from build123d import *

# Parameters (mm, degrees)
CORTAR_EXTRUIR1_DEPTH = 15


with BuildPart() as part:
    # Croquis1 → Revolución1 (revolve)
    with BuildSketch(Plane(origin=(0, 0, 0), x_dir=(0, 0, -1), z_dir=(1, 0, 0))):
        Polygon((40, 10), (0, 10), (0, -10), (40, -10), (40, -4.682903261), (36.75, -3.5), (36.75, 3.5), (40, 4.682903261), align=None)
    revolve(axis=Axis((0, 0, 0), (0, 1, 0)))

    # Croquis2 → Cortar-Extruir1 (cut, symmetric)
    with BuildSketch(Plane(origin=(0, 0, 0), x_dir=(1, 0, 0), z_dir=(0, 1, 0))):
        with BuildLine():
            Line((3, 2.645751311), (3, -2.645751311))
            ThreePointArc((3, -2.645751311), (-4, 0), (3, 2.645751311))
        make_face()
    extrude(amount=CORTAR_EXTRUIR1_DEPTH, both=True, mode=Mode.SUBTRACT)


solid = part.part
The model under review builds one solid part; all positions refer to its coordinate system, in mm. A direction names the side the tool comes from. Round coordinates to 2 decimals unless told otherwise and drop trailing zeros. Order: outer loops, then holes, each group sorted by start corner. A loop starts at its lowest first (then second) coordinate and runs counter-clockwise, first axis right, second up. Notation, with made-up numbers: (1, 27.5) - (33, 27.5) arc R6 ccw to (33, 31.5) - close; hole circle Ø2 at (17.25, -12). An arc over 180 degrees is marked (long way). Use one line per item in the form item = value.
Q1. Add section D-D on y = -1.5. Give the boundary of the cut face in (x, z), then the cut area to 3 significant figures.
Response values:
outline = circle Ø73.5 at (0, 0); hole (3, -2.65) - (3, 2.65) arc R4 ccw (long way) to start
area = 4,200 mm^2
Q2. Tool access review of faces 4 (the flat face through (-1, -10, 8)), 5 (the cylindrical face through (35.876, 0.049, 7.967)), 6 (the flat face through (3, 0, 0)): name each direction out of +Z, -Z, +X, -X, +Y, -Y from which nothing blocks a thin tool from reaching the whole face with its end or side.
Response values:
face_4 = +Z, -Z, +X, -X, -Y
face_5 = none
face_6 = +Y, -Y
Q3. To check wall thickness, follow line 1 (Z direction, x = 0, y = -5.5); line 2 (X direction, y = 5, z = 0); line 3 (X direction, y = 2, z = 0). State the ranges of each line that lie inside material, in increasing order.
Response values:
line_1 = -40 to -4, 4 to 40
line_2 = -40 to -4, 3 to 40
line_3 = -36.75 to -4, 3 to 36.75
Q4. Add section C-C on y = 8. Give the boundary of the cut face in (x, z).
Response values:
outline = circle Ø80 at (0, 0); hole (3, -2.65) - (3, 2.65) arc R4 ccw (long way) to start
Q5. Add section B-B on x = 0. Give the boundary of the cut face in (y, z).
Response values:
outline = (-10, -40) - (-4.68, -40) - (-3.5, -36.75) - (3.5, -36.75) - (4.68, -40) - (10, -40) - (10, -4) - (-10, -4) - close; (-10, 4) - (10, 4) - (10, 40) - (4.68, 40) - (3.5, 36.75) - (-3.5, 36.75) - (-4.68, 40) - (-10, 40) - close
Q6. Mouldability with a two-part tool opening along Y and no side actions: class faces 1 (the cylindrical face through (-4, 0, 0)), 2 (the flat face through (-1, 10, -8)), 3 (the conical face through (36.075, 3.574, 8.011)) as pulls with the +Y half, pulls with the -Y half, needs draft (parallel to the pull), parting line crosses it, or undercut.
Response values:
face_1 = needs draft
face_2 = pulls with the +Y half
face_3 = undercut
Q7. Add section A-A on z = 0. Give the boundary of the cut face in (x, y), then the cut area to 3 significant figures.
Response values:
outline = (-40, -10) - (-4, -10) - (-4, 10) - (-40, 10) - (-40, 4.68) - (-36.75, 3.5) - (-36.75, -3.5) - (-40, -4.68) - close; (3, -10) - (40, -10) - (40, -4.68) - (36.75, -3.5) - (36.75, 3.5) - (40, 4.68) - (40, 10) - (3, 10) - close
area = 1,410 mm^2
Q8. Clearance check with flat-ended pins moving along their axes: P1, Ø2, axis at y = 6.5, z = -9, coming from the +X side; P2, Ø12, axis at x = -2, y = -0.5, coming from the -Z side; P3, Ø12, axis at x = 10.5, y = -1.5, coming from the +Z side; P4, Ø10, axis at x = 14, y = -1.5, coming from the -Z side. State where each tip first meets the part, or that it passes through.
Response values:
P1 = 39.19
P2 = -40
P3 = 39.63
P4 = -38.69
